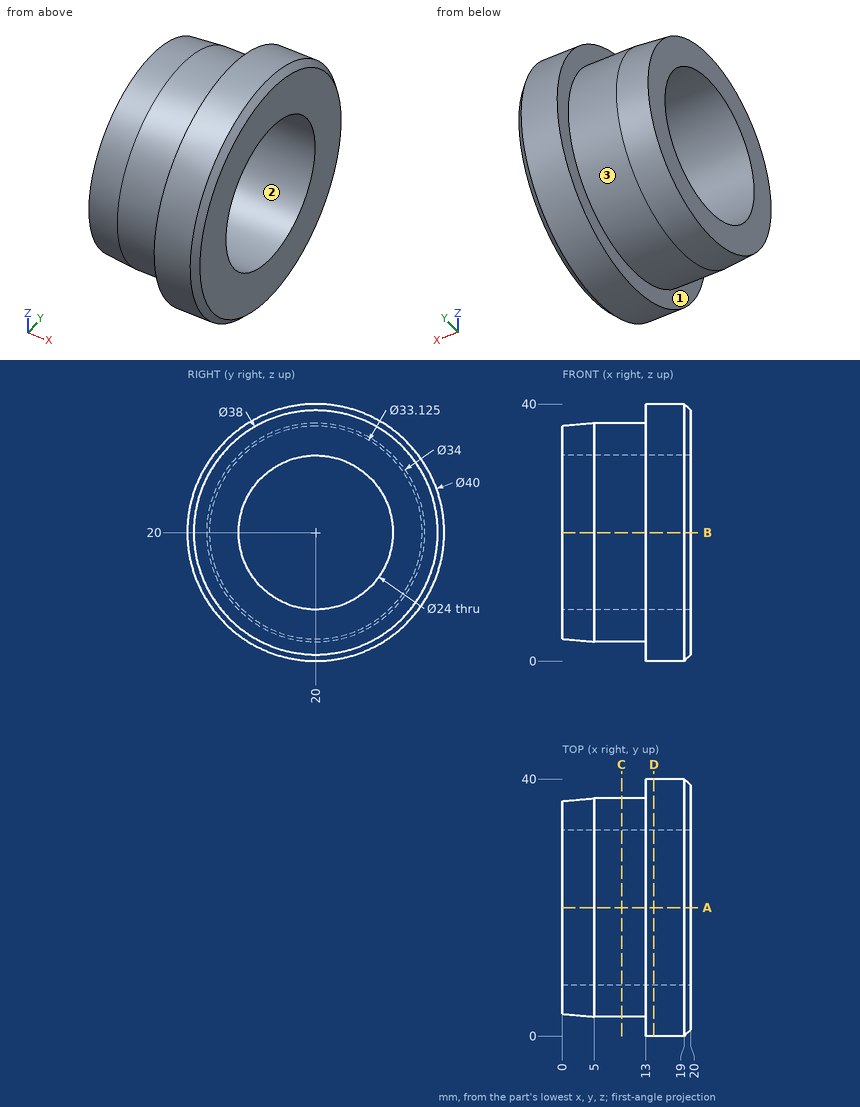
Print and shaded views of the part. All mm, measured from the part's lowest x, y and z. Give positions to 0.01 mm unless a question says otherwise; leave off trailing zeros. Loops run counter-clockwise (first coordinate to the right, second up) from the corner with the lowest first, then second, coordinate; pieces in that order, holes last. Notation, with made-up numbers: (38.5, 14.5) - (89.5, 14.5) arc R17 cw to (89.5, 47.5) - close; hole circle Ø4 at (74, -27.5). An arc over 180 degrees is marked (long way). One line per item, written item: value. Start each with the question number.
1. Slice it at D-D (x = 14.25). List the corners of the cut face in (y, z), plus the area to 3 significant figures.
2. Slice it at A-A (y = 20). List the corners of the cut face in (x, z), plus the area to 3 significant figures.
3. Pin check, flat tips, straight feed: pin 1 (1.5 mm diameter, centred on x = 3, y = 27.5, fed in from -Z); pin 2 (4 mm diameter, centred on x = 13.5, y = 16, fed in from +Z); pin 3 (4 mm diameter, centred on x = 17, y = 35, fed in from +Z); pin 4 (10 mm diameter, centred on x = 8.5, y = 18.5, fed in from +Z). Stop position of each tip, or through.
4. Probe L1, parallel to Z at x = 7.5, y = 20; L2, parallel to Y at x = 14, z = 22.5; L3, parallel to X at y = 30.5, z = 5.5. List the from-to ranges inside material, lowest first. Write a range as from..to.
5. Slice it at C-C (x = 9.25). List the corners of the cut face in (y, z).
6. Pull direction Y, two halves, no side cores. Call the marked faces 1, 2 and 3: pulls with the +Y half, pulls with the -Y half, needs draft (parallel to the pull), parting line crosses it, or undercut.
Solution:
1. outline: circle Ø40 at (20, 20); hole circle Ø24 at (20, 20)
1. area: 804 mm^2
2. outline: (0, 3.44) - (5, 3) - (13, 3) - (13, 0) - (19, 0) - (20, 1) - (20, 8) - (0, 8) - close; (0, 32) - (20, 32) - (20, 39) - (19, 40) - (13, 40) - (13, 37) - (5, 37) - (0, 36.56) - close
2. area: 239 mm^2
3. pin 1: stops at z = 4.58
3. pin 2: stops at z = 39.9
3. pin 3: stops at z = 35.2
3. pin 4: stops at z = 40
4. L1: z = 3..8, 32..37
4. L2: y = 0.16..8.26, 31.74..39.84
4. L3: x = 13..20
5. outline: circle Ø34 at (20, 20); hole circle Ø24 at (20, 20)
6. face 1: needs draft
6. face 2: undercut
6. face 3: parting line crosses it
